Can you work these out from the drawing? Everything is in mm from the part's minimum corner. Give positions to 0.01 mm unless a question says otherwise; leave off trailing zeros. Order: outer loops, then holes, each group sorted by start corner. A loop starts at its lowest first (then second) coordinate and runs counter-clockwise, first axis right, second up. Notation, with made-up numbers: (50, 54) - (97, 54) arc R23 ccw to (97, 69) - close; hole circle Ø5 at (10, 54.5). An arc over 180 degrees is marked (long way). Answer as a JSON object with one key per item and string values.
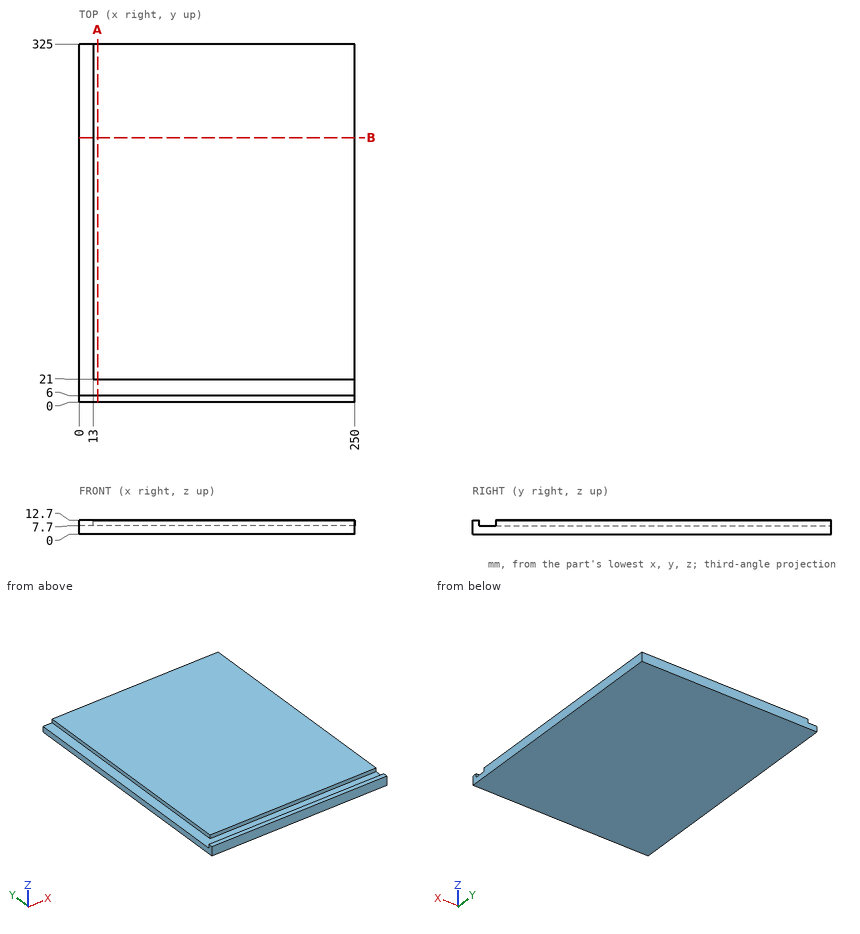
Q1. If we section it at A-A, the plane x = 17: Please give me the cut outline in (y, z), then the cut area to 3 significant figures.
Recorded:
{"outline": "(0, 0) - (325, 0) - (325, 12.7) - (21, 12.7) - (21, 7.7) - (6, 7.7) - (6, 12.7) - (0, 12.7) - close", "area": "4,050 mm^2"}
Q2. I need wall thicknesses on L1, parallel to Y at x = 132, z = 11.5; L2, parallel to X at y = 288.5, z = 11.5. Which ranges of each line are inside material? Lowest first, please.
Recorded:
{"L1": "y = 0 to 6, 21 to 325", "L2": "x = 13 to 250"}
Q3. I'm going to push a flat-ended pin straight in: pin 1 Ø2.5 at (y, z) = (238, 9.5) entering from -X. Where does the tip first touch, or does it pass through?
Recorded:
{"pin 1": "stops at x = 13"}
Q4. If we section it at B-B, the plane y = 240: Please give me the cut outline in (x, z), then the cut area to 3 significant figures.
Recorded:
{"outline": "(0, 0) - (250, 0) - (250, 12.7) - (13, 12.7) - (13, 7.7) - (0, 7.7) - close", "area": "3,110 mm^2"}
